Input: part model. Units: mm. Frame: model coordinates. Coordinates: 2 decimals unless noted, no trailing zeros. Order: outer loops, then holes, each group sorted by start corner. A loop starts at its lowest first (then second) coordinate and runs counter-clockwise, first axis right, second up. Notation, with made-up numbers: (-31.75, -1.75) -> (-2.75, -1.75) arc R27 ccw to (-2.75, 33.25) -> close; hole circle Ø4 at (71.25, -37.75). An arc over 180 degrees is marked (long way). Use one line per item in the form item = value. Start each with the question number.
1) Section query A-A on z = -17. Output: boundary loops of the cut face in (x, y), then the cut area to 4 significant figures.
2) Section query C-C on x = 25.5. Output: boundary loops of the cut face in (y, z).
3) Section query D-D on z = 1. Output: boundary loops of the cut face in (x, y).
4) Section query B-B on y = -3. Count the separate pieces of the cut face and the enclosed holes in it, then the cut area to 3 significant figures.
5) Pin query (flat end, axial travel): pin 1 (0.8 mm diameter, centred on x = -39.5, y = -4, fed in from +Z); pin 2 (1.2 mm diameter, centred on y = -4, z = 33, fed in from +X); pin 3 (1.5 mm diameter, centred on y = -9, z = -12.5, fed in from -X). Return the tip coordinate at first contact, or that it passes through.
6) Draft query along Z for faces 1 (the cylindrical face through (44.858, -5.07, -19.578)), 2 (the cylindrical face through (32.01, -4.93, 25.35)), 3 (the flat face through (0, -6, -36)). Return one class per face: pulls with the +Z half, pulls with the -Z half, needs draft (parallel to the pull), parting line crosses it, or undercut.
7) Ray query, line 1 along Z through (x, y) = (25.5, -6.25); line 2 along X through (y, z) = (-2.75, 17); line 3 along Z through (x, y) = (-25, -7). Return the intervals inside material, ascending.
from build123d import *

# Parameters (mm, degrees)
BOSS_EXTRUDE1_DEPTH        = 10
SKETCH2_W                  = 58
SKETCH2_H                  = 10
BOSS_EXTRUDE2_DEPTH        = 13.5
SKETCH3_W                  = 58
SKETCH3_H                  = 10
BOSS_EXTRUDE3_DEPTH        = 13.5
F_4_0_4_DIAMETER_HOLE1_D   = 4
F_3_9_3_9_DIAMETER_HOLE1_D = 3.9
CHAMFER1_SIZE              = 1.5
CHAMFER2_SIZE              = 2
FILLET1_R                  = 10


with BuildPart() as part:
    # Sketch1 → Boss-Extrude1 (new body)
    with BuildSketch(Plane.XZ.offset(10)):
        with BuildLine():
            Line((-40, -22.5), (40, -22.5))
            ThreePointArc((40, -22.5), (44.897390752, -19.503110829), (44.457713391, -13.778386844))
            ThreePointArc((44.457713391, -13.778386844), (40, 0), (44.457713391, 13.778386844))
            ThreePointArc((44.457713391, 13.778386844), (44.897390752, 19.503110829), (40, 22.5))
            Line((40, 22.5), (-40, 22.5))
            ThreePointArc((-40, 22.5), (-44.897390752, 19.503110829), (-44.457713391, 13.778386844))
            ThreePointArc((-44.457713391, 13.778386844), (-40, 0), (-44.457713391, -13.778386844))
            ThreePointArc((-44.457713391, -13.778386844), (-44.897390752, -19.503110829), (-40, -22.5))
        make_face()
    extrude(amount=-BOSS_EXTRUDE1_DEPTH)

    # Sketch2 → Boss-Extrude2 (add)
    with BuildSketch(Plane(origin=(0, 0, -22.5), x_dir=(-1, 0, 0), z_dir=(0, 0, -1))):
        with Locations((0, -5)):
            Rectangle(SKETCH2_W, SKETCH2_H)
    extrude(amount=BOSS_EXTRUDE2_DEPTH)

    # Sketch3 → Boss-Extrude3 (add)
    with BuildSketch(Plane.XY.offset(22.5)):
        with Locations((0, -5)):
            Rectangle(SKETCH3_W, SKETCH3_H)
    extrude(amount=BOSS_EXTRUDE3_DEPTH)

    # Ø4.0 (4) Diameter Hole1 (through all)
    with Locations(Plane(origin=(0, 0, 0), x_dir=(1, 0, 0), z_dir=(0, 1, 0))):
        with Locations((-25.5, -17), (-25.5, 17), (25.5, 17), (25.5, -17)):
            Hole(F_4_0_4_DIAMETER_HOLE1_D / 2)

    # Ø3.9 (3.9) Diameter Hole1 (through all)
    with Locations(Plane(origin=(0, -10, 0), x_dir=(-1, 0, 0), z_dir=(0, -1, 0))):
        with Locations((40, 17), (-40, 17), (-40, -17), (40, -17)):
            Hole(F_3_9_3_9_DIAMETER_HOLE1_D / 2)

    # Chamfer1
    chamfer1_edges = [part.edges().sort_by_distance(p)[0] for p in [
        (-41.95, -10, 17),
        (38.05, -10, 17),
        (38.05, -10, -17),
        (-41.95, -10, -17),
    ]]
    chamfer(chamfer1_edges, length=CHAMFER1_SIZE)

    # Chamfer2
    chamfer2_edges = [part.edges().sort_by_distance(p)[0] for p in [
        (-29, -5, -36),
        (0, 0, -36),
        (29, -5, -36),
        (29, -5, 36),
        (0, 0, 36),
        (-29, -5, 36),
    ]]
    chamfer(chamfer2_edges, length=CHAMFER2_SIZE)

    # Fillet1
    fillet1_edges = [part.edges().sort_by_distance(p)[0] for p in [
        (-29, -5, -22.5),
        (29, -5, -22.5),
        (29, -5, 22.5),
        (-29, -5, 22.5),
    ]]
    fillet(fillet1_edges, radius=FILLET1_R)


solid = part.part
Answers below:
q1.outline = (-45.5, -10) -> (-43.45, -10) -> (-41.95, -8.5) -> (-41.95, 0) -> (-45.5, 0) -> close; (-38.05, -8.5) -> (-36.55, -10) -> (-27.5, -10) -> (-27.5, 0) -> (-38.05, 0) -> close; (-23.5, -10) -> (23.5, -10) -> (23.5, 0) -> (-23.5, 0) -> close; (27.5, -10) -> (36.55, -10) -> (38.05, -8.5) -> (38.05, 0) -> (27.5, 0) -> close; (41.95, -8.5) -> (43.45, -10) -> (45.5, -10) -> (45.5, 0) -> (41.95, 0) -> close
q1.area = 747.5 mm^2
q2.outline = (-10, -36) -> (-2, -36) -> (0, -34) -> (0, -19) -> (-10, -19) -> close; (-10, -15) -> (0, -15) -> (0, 15) -> (-10, 15) -> close; (-10, 19) -> (0, 19) -> (0, 34) -> (-2, 36) -> (-10, 36) -> close
q3.outline = (-40.02, -10) -> (40.02, -10) -> (40.02, 0) -> (-40.02, 0) -> close
q4.separate_pieces = 1
q4.enclosed_holes = 8
q4.area = 5,390 mm^2
q5.pin_1 = 22.5
q5.pin_2 = 29
q5.pin_3 = -44.09
q6.face_1 = undercut
q6.face_2 = pulls with the +Z half
q6.face_3 = pulls with the -Z half
q7.line_1 = -36 to -19, -15 to 15, 19 to 36
q7.line_2 = -45.5 to -41.95, -38.05 to -27.5, -23.5 to 23.5, 27.5 to 38.05, 41.95 to 45.5
q7.line_3 = -36 to -18.94, -15.06 to 15.06, 18.94 to 36
